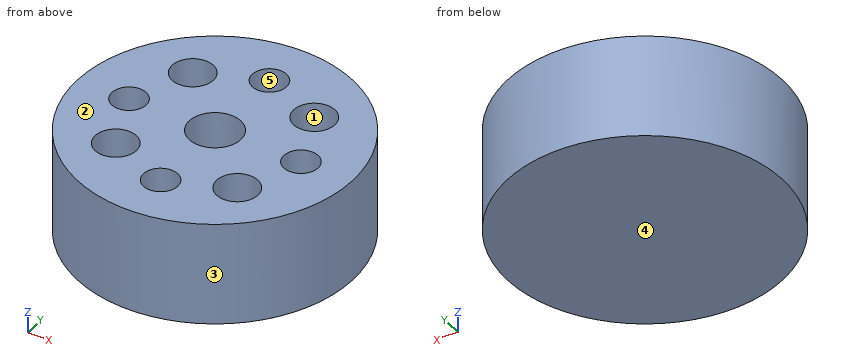
```python
from build123d import *

# Parameters (mm, degrees)
SKIZZE1_R                       = 40
AUFSATZ_LINEAR_AUSTRAGEN1_DEPTH = 30
SKIZZE2_R                       = 5
SCHNITT_LINEAR_AUSTRAGEN1_DEPTH = 25
SKIZZE4_R                       = 6
SCHNITT_LINEAR_AUSTRAGEN5_DEPTH = 25
SKIZZE5_R                       = 7.5
SCHNITT_LINEAR_AUSTRAGEN6_DEPTH = 25


with BuildPart() as part:
    # Skizze1 → Aufsatz-Linear austragen1 (new body)
    with BuildSketch(Plane.XY):
        Circle(SKIZZE1_R)
    extrude(amount=AUFSATZ_LINEAR_AUSTRAGEN1_DEPTH)

    # Skizze2 → Schnitt-Linear austragen1 (cut)
    with BuildSketch(Plane.XY.offset(30)):
        with Locations((25, 0)):
            Circle(SKIZZE2_R)
        with Locations((0, -25)):
            Circle(SKIZZE2_R)
        with Locations((-25, 0)):
            Circle(SKIZZE2_R)
        with Locations((0, 25)):
            Circle(SKIZZE2_R)
    extrude(amount=-SCHNITT_LINEAR_AUSTRAGEN1_DEPTH, mode=Mode.SUBTRACT)

    # Skizze4 → Schnitt-Linear austragen5 (cut)
    with BuildSketch(Plane.XY.offset(30)):
        with Locations((17.67766953, 17.67766953)):
            Circle(SKIZZE4_R)
        with Locations((17.67766953, -17.67766953)):
            Circle(SKIZZE4_R)
        with Locations((-17.67766953, -17.67766953)):
            Circle(SKIZZE4_R)
        with Locations((-17.67766953, 17.67766953)):
            Circle(SKIZZE4_R)
    extrude(amount=-SCHNITT_LINEAR_AUSTRAGEN5_DEPTH, mode=Mode.SUBTRACT)

    # Skizze5 → Schnitt-Linear austragen6 (cut)
    with BuildSketch(Plane.XY.offset(30)):
        Circle(SKIZZE5_R)
    extrude(amount=-SCHNITT_LINEAR_AUSTRAGEN6_DEPTH, mode=Mode.SUBTRACT)


solid = part.part
```
Check sheet for the modelled part. Datum: model origin and axes. Units: mm. Face numbers are marked on the shaded views. A direction names the side the tool comes from. Coordinates: 2 decimals unless noted, no trailing zeros. Write each loop counter-clockwise with the first axis right and the second up, starting at its lowest first coordinate (ties: lowest second). Pieces come first, ordered by that corner, then holes. Notation, with made-up numbers: M 24,20.25 L 60,20.25 A31 ccw 60,47.25 Z; hole C -9,41.25 d1. An arc over 180 degrees is marked long. Use one line per item in the form item = value.
Item 1: Release check for a two-part mould opening along Y. For the marked faces 3, 4 and 5 record: pulls with the +Y half, pulls with the -Y half, needs draft (parallel to the pull), parting line crosses it, or undercut.
Answer below:
face_3 = parting line crosses it
face_4 = needs draft
face_5 = undercut
Item 2: Set-up check for the marked faces 1 and 2: record each of +Z, -Z, +X, -X, +Y, -Y from which the full face is reachable in a straight line by a thin tool's end or side.
Answer below:
face_1 = +Z
face_2 = +Z, +X, -X, +Y, -Y
Item 3: Sectioned sample at A-A, the plane x = 0. Record the cut outline in (y, z).
Answer below:
outline = M -40,0 L 40,0 L 40,30 L 30,30 L 30,5 L 20,5 L 20,30 L 7.5,30 L 7.5,5 L -7.5,5 L -7.5,30 L -20,30 L -20,5 L -30,5 L -30,30 L -40,30 Z
Item 4: Sectioned sample at B-B, the plane z = 26.25. State how many separate pieces and enclosed holes the cut face has, and give its area (3 significant figures).
Answer below:
separate_pieces = 1
enclosed_holes = 9
area = 4,080 mm^2
Item 5: Sectioned sample at C-C, the plane y = -25. Record the cut outline in (x, z), and give its area (3 significant figures).
Answer below:
outline = M -31.22,0 L 31.22,0 L 31.22,30 L 5,30 L 5,5 L -5,5 L -5,30 L -31.22,30 Z
area = 1,620 mm^2
Item 6: Gauge pin test, flat ends, axial feed: pin 1 Ø11 at (x, y) = (-17.68, 17.68) entering from +Z; pin 2 Ø8 at (y, z) = (8, 20) entering from +X; pin 3 Ø1.5 at (x, z) = (21.5, 24) entering from -Y. Record the tip position at first contact, or that the pin passes through.
Answer below:
pin_1 = 5
pin_2 = 39.8
pin_3 = -34.2
Item 7: Material ranges on L1, parallel to Y at x = -19, z = 16.5; L2, parallel to X at y = -4.5, z = 22; L3, parallel to X at y = 19.5, z = 10.75, recorded low to high. Write a range as from..to.
Answer below:
L1 = -35.2..-23.53, -11.83..11.83, 23.53..35.2
L2 = -39.75..-27.18, -22.82..-6, 6..22.82, 27.18..39.75
L3 = -34.92..-23.39, -11.96..11.96, 23.39..34.92
